Here's how the part is built. I have some questions about the finished solid (model axes, mm). Round coordinates to 2 decimals unless told otherwise and drop trailing zeros. Order: outer loops, then holes, each group sorted by start corner. A loop starts at its lowest first (then second) coordinate and runs counter-clockwise, first axis right, second up. Notation, with made-up numbers: M 61.5,32 L 79.5,32 A31 cw 79.5,60 Z; hole C 19.5,-0.75 d11. An arc over 180 degrees is marked long. Write item = value, one per line. Start each with the question number.
Item 1: I want a section at C-C, the plane x = 6. List the corners of the cut face in (y, z) for me.
Item 2: I want a section at A-A, the plane y = 0. List the corners of the cut face in (x, z) for me (3 decimals).
Item 3: I'm going to push flat-ended pins straight in: P1, Ø1, axis at x = 12, y = -15, coming from the -Z side; P2, Ø8, axis at x = 10, z = -13, coming from the +Y side; P3, Ø6, axis at x = 2, y = -1.5, coming from the -Z side. Where does each tip first touch, or does it pass through?
Item 4: Please list where these lines run through material, in increasing order: L1, parallel to Z at x = 13.25, y = -0.5; L2, parallel to Y at x = 12.5, z = -23.5; L3, parallel to Y at x = 3.75, z = -7.
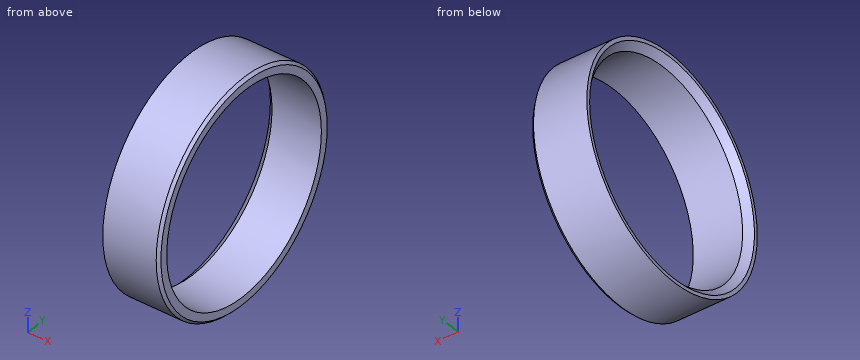
```python
from build123d import *

# Parameters (mm, degrees)
F0_R     = 32
F0_R_2   = 29.05
F1_DEPTH = 15.875
F2_SIZE  = 1.905
F3_SIZE  = 0.762


with BuildPart() as f1:
    # F0 (on Right) → F1 (new body)
    with BuildSketch(Plane.YZ):
        Circle(F0_R)
        Circle(F0_R_2, mode=Mode.SUBTRACT)
    extrude(amount=F1_DEPTH)

    # F2
    f2_edges = [f1.edges().sort_by_distance(p)[0] for p in [
        (0, -29.05, 0),
    ]]
    chamfer(f2_edges, length=F2_SIZE)

    # F3
    f3_edges = [f1.edges().sort_by_distance(p)[0] for p in [
        (15.875, -32, 0),
    ]]
    chamfer(f3_edges, length=F3_SIZE)


solid = f1.part
```
Filled in:
q1.outline = C 0,0 d64; hole C 0,0 d58.1
q2.outline = M 0,-32 L 15.113,-32 L 15.875,-31.238 L 15.875,-29.05 L 1.905,-29.05 L 0,-30.955 Z; M 0,30.955 L 1.905,29.05 L 15.875,29.05 L 15.875,31.238 L 15.113,32 L 0,32 Z
q3.P1 = -28.53
q3.P2 = 30.71
q3.P3 = -32
q4.L1 = -32 to -29.05, 29.05 to 32
q4.L2 = -21.72 to -17.08, 17.08 to 21.72
q4.L3 = -31.22 to -28.19, 28.19 to 31.22
